from build123d import *

# Parameters (mm, degrees)
SKETCH1_R           = 73.66
BOSS_EXTRUDE1_DEPTH = 12.7
SKETCH2_R           = 2
CUT_EXTRUDE1_DEPTH  = 12.7
SKETCH3_R           = 66
SKETCH3_R_2         = 65
BOSS_EXTRUDE2_DEPTH = 88.9
SKETCH4_R           = 65
SKETCH4_R_2         = 28.162552898
BOSS_EXTRUDE3_DEPTH = 3
SKETCH5_R           = 65
SKETCH5_R_2         = 28.162552898
BOSS_EXTRUDE4_DEPTH = 3
CUT_EXTRUDE2_START  = -300
SKETCH6_R           = 28.162552898
CUT_EXTRUDE2_DEPTH  = 300


with BuildPart() as part:
    # Sketch1 → Boss-Extrude1 (new body)
    with BuildSketch(Plane.XY):
        Circle(SKETCH1_R)
    extrude(amount=BOSS_EXTRUDE1_DEPTH)

    # Sketch2 → Cut-Extrude1 (cut)
    with BuildSketch(Plane.XY.offset(12.7)):
        with Locations((0, 69)):
            Circle(SKETCH2_R)
        with Locations((34.5, 59.755752861)):
            Circle(SKETCH2_R)
        with Locations((59.755752861, 34.5)):
            Circle(SKETCH2_R)
        with Locations((69, 0)):
            Circle(SKETCH2_R)
        with Locations((59.755752861, -34.5)):
            Circle(SKETCH2_R)
        with Locations((34.5, -59.755752861)):
            Circle(SKETCH2_R)
        with Locations((0, -69)):
            Circle(SKETCH2_R)
        with Locations((-34.5, -59.755752861)):
            Circle(SKETCH2_R)
        with Locations((-59.755752861, -34.5)):
            Circle(SKETCH2_R)
        with Locations((-69, 0)):
            Circle(SKETCH2_R)
        with Locations((-59.755752861, 34.5)):
            Circle(SKETCH2_R)
        with Locations((-34.5, 59.755752861)):
            Circle(SKETCH2_R)
    extrude(amount=-CUT_EXTRUDE1_DEPTH, mode=Mode.SUBTRACT)

    # Sketch3 → Boss-Extrude2 (add)
    with BuildSketch(Plane.XY.offset(12.7)):
        Circle(SKETCH3_R)
        Circle(SKETCH3_R_2, mode=Mode.SUBTRACT)
    extrude(amount=BOSS_EXTRUDE2_DEPTH)

    # Sketch4 → Boss-Extrude3 (add)
    with BuildSketch(Plane.XY.offset(32.7)):
        Circle(SKETCH4_R)
        Circle(SKETCH4_R_2, mode=Mode.SUBTRACT)
    extrude(amount=BOSS_EXTRUDE3_DEPTH)

    # Sketch5 → Boss-Extrude4 (add)
    with BuildSketch(Plane.XY.offset(55.7)):
        Circle(SKETCH5_R)
        Circle(SKETCH5_R_2, mode=Mode.SUBTRACT)
    extrude(amount=BOSS_EXTRUDE4_DEPTH)

    # Sketch6 → Cut-Extrude2 (cut)
    with BuildSketch(Plane.XY.offset(12.7).offset(CUT_EXTRUDE2_START)):
        Circle(SKETCH6_R)
    extrude(amount=CUT_EXTRUDE2_DEPTH, mode=Mode.SUBTRACT)


solid = part.part
Part model, mm, in its own coordinate system. A direction names the side the tool comes from. Coordinates: 2 decimals unless noted, no trailing zeros. Loops run counter-clockwise (first coordinate to the right, second up) from the corner with the lowest first, then second, coordinate; pieces in that order, holes last. Notation, with made-up numbers: (22.5, 25) - (49.5, 25) arc R16 ccw to (49.5, 51) - close; hole circle Ø8 at (48.25, 19). An arc over 180 degrees is marked (long way). Write each question's results on one line, items separated by ' | '. Start each with the question number.
Q1. Slice it at C-C on x = -47. Give the cut face in (y, z).
Q2. Two-plate mould, pull along Y, no slides. Class faces 4 (the cylindrical face through (36.347, 58.99, 6.439)), 5 (the flat face through (48.6, -43.7, 101.6)): +Y half, -Y half, draft (parallel to the pull), parting line (faces both ways), or undercut.
Q3. Slice it at A-A on x = 34.5. Give the cut face in (y, z) (3 decimals).
Q4. Drop flat-ended pins along their axis: pin 1 Ø12 at (y, z) = (7, 24) entering from +X; pin 2 Ø4.5 at (x, y) = (0, 69) entering from +Z; pin 3 Ø6 at (x, z) = (-51, 39) entering from -Y. Give the stop position or say it passes through.
Q5. Slice it at D-D on z = 41. Give the cut face in (x, y).
Q6. Probe line 1 along Z through (x, y) = (24, -37); line 2 along Y through (x, z) = (0, 4); line 3 along X through (y, z) = (2, 29). List the from-to ranges inside material, lowest first.
Q7. Which spindle directions (+Z, -Z, +X, -X, +Y, -Y) get a long thin tool onto all of the face, cutting with end or side? Do faces 1 (the cylindrical face through (62, 19.52, 79.85)), 2 (the cylindrical face through (62, 19.52, 22.56)), 3 (the cylindrical face through (-22.349, -17.136, 34.179)). Say none if no direction does.
Answer:
1) outline: (-56.72, 0) - (56.72, 0) - (56.72, 12.7) - (46.34, 12.7) - (46.34, 101.6) - (44.9, 101.6) - (44.9, 58.7) - (-44.9, 58.7) - (-44.9, 101.6) - (-46.34, 101.6) - (-46.34, 12.7) - (-56.72, 12.7) - close; hole (-44.9, 12.7) - (44.9, 12.7) - (44.9, 32.7) - (-44.9, 32.7) - close; hole (-44.9, 35.7) - (44.9, 35.7) - (44.9, 55.7) - (-44.9, 55.7) - close
2) face 4: undercut | face 5: draft
3) outline: (-65.081, 0) - (-61.756, 0) - (-61.756, 12.7) - (-65.081, 12.7) - close; (-57.756, 0) - (57.756, 0) - (57.756, 12.7) - (56.265, 12.7) - (56.265, 101.6) - (55.089, 101.6) - (55.089, 58.7) - (-55.089, 58.7) - (-55.089, 101.6) - (-56.265, 101.6) - (-56.265, 12.7) - (-57.756, 12.7) - close; (61.756, 0) - (65.081, 0) - (65.081, 12.7) - (61.756, 12.7) - close; hole (-55.089, 12.7) - (55.089, 12.7) - (55.089, 32.7) - (-55.089, 32.7) - close; hole (-55.089, 35.7) - (55.089, 35.7) - (55.089, 55.7) - (-55.089, 55.7) - close
4) pin 1: stops at x = 65.99 | pin 2: stops at z = 12.7 | pin 3: stops at y = -45.3
5) outline: circle Ø132 at (0, 0); hole circle Ø130 at (0, 0)
6) line 1: z = 0 to 12.7, 32.7 to 35.7, 55.7 to 58.7 | line 2: y = -73.66 to -71, -67 to -28.16, 28.16 to 67, 71 to 73.66 | line 3: x = -65.97 to -64.97, 64.97 to 65.97
7) face 1: +Z | face 2: none | face 3: +Z, -Z
